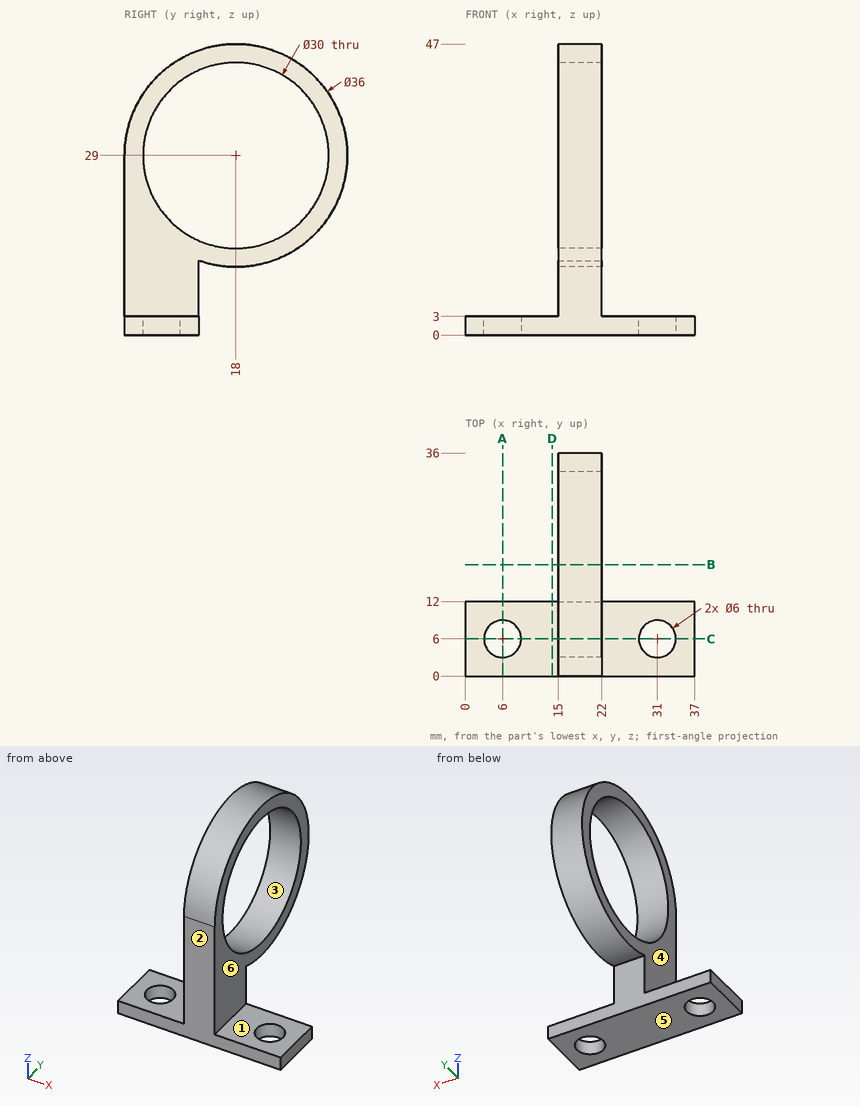
Verification items for this drawing (mm, ordinates from the low corner). A direction names the side the tool comes from. Coordinates: 2 decimals unless noted, no trailing zeros. Write each loop counter-clockwise with the first axis right and the second up, starting at its lowest first coordinate (ties: lowest second). Pieces come first, ordered by that corner, then holes. Notation, with made-up numbers: M 61.5,-28.5 L 83.5,-28.5 A24 ccw 83.5,-16.5 Z; hole C 46.25,6 d10. An arc over 180 degrees is marked long. Answer as a JSON object with one key per item and string values. Group by question number.
(1) Cross-section at C-C, the plane y = 6. Record the cut outline in (x, z), and give its area (3 significant figures).
(2) Tool access check on the marked faces 4, 5 and 6. Record the directions out of +Z, -Z, +X, -X, +Y, -Y that give a thin tool (end or side, any length) a straight path to the whole face; none if there is none.
(3) Gauge pin test, flat ends, axial feed: pin 1 (18 mm diameter, centred on y = 25, z = 20.5, fed in from +X); pin 2 (6 mm diameter, centred on x = 4.5, y = 6, fed in from +Z); pin 3 (6 mm diameter, centred on x = 13.5, z = 3.5, fed in from +Y). Record the tip position at first contact, or that the pin passes through.
(4) Release check for a two-part mould opening along Y. For the marked faces 1, 2 and 3 record: +Y half, -Y half, draft (parallel to the pull), parting line (faces both ways), or undercut.
(5) Cross-section at B-B, the plane y = 18. Record the cut outline in (x, z), and give its area (3 significant figures).
(6) Cross-section at A-A, the plane x = 6. Record the cut outline in (y, z), and give its area (3 significant figures).
(7) Material ranges on line 1 (Y direction, x = 6, z = 1.7); line 2 (Z direction, x = 18, y = 18); line 3 (X direction, y = 5.5, z = 5), recorded low to high.
(8) Cross-section at D-D, the plane x = 14. Record the cut outline in (y, z).
Reply:
{
 "1": {"outline": "M 0,0 L 3,0 L 3,3 L 0,3 Z; M 9,0 L 28,0 L 28,3 L 22,3 L 22,20 L 15,20 L 15,3 L 9,3 Z; M 15,38 L 22,38 L 22,42.42 L 15,42.42 Z; M 34,0 L 37,0 L 37,3 L 34,3 Z", "area": "225 mm²"},
 "2": {"face 4": "+Z, -X, +Y, -Y", "face 5": "-Z, +X, -X, +Y, -Y", "face 6": "+Z, +X, +Y, -Y"},
 "3": {"pin 1": "x = 22", "pin 2": "z = 3", "pin 3": "y = 12"},
 "4": {"face 1": "draft", "face 2": "-Y half", "face 3": "undercut"},
 "5": {"outline": "M 15,11 L 22,11 L 22,14 L 15,14 Z; M 15,44 L 22,44 L 22,47 L 15,47 Z", "area": "42.0 mm²"},
 "6": {"outline": "M 0,0 L 3,0 L 3,3 L 0,3 Z; M 9,0 L 12,0 L 12,3 L 9,3 Z", "area": "18.0 mm²"},
 "7": {"line 1": "0 to 3, 9 to 12", "line 2": "11 to 14, 44 to 47", "line 3": "15 to 22"},
 "8": {"outline": "M 0,0 L 12,0 L 12,3 L 0,3 Z"}
}
